Can you work these out from the model? Positions are in its coordinate system, mm. Round coordinates to 2 decimals unless told otherwise and drop trailing zeros. Answer in a Markdown table with one row per item. Add a question column.
(1) Suppose I cut it at A-A, the plane y = -7. Count the separate pieces of the cut face and the enclosed holes in it, then the cut area to 3 significant figures.
(2) If we mould it in two halves opening along X, with no side actions, what happens to faces 1 (the face through (-8.4, 7.8, 7)), 2 (the face through (-0.13, -14.96, 3.48))? For each: released by +X, released by -X, zero draft, split by the parting line, or undercut.
(3) I'm going to push flat-ended pins straight in: pin 1 (4 mm diameter, centred on y = 10, z = 6, fed in from +X); pin 2 (6 mm diameter, centred on x = -1.5, y = 6.5, fed in from +Z); pin 3 (4 mm diameter, centred on x = 16, z = 3.5, fed in from -Y); pin 4 (2 mm diameter, centred on y = -1.5, z = 2.5, fed in from -X). Where does each tip first touch, or does it pass through?
(4) If I drill on probe 1 along Y at (x, z) = (-24, 4.75) (3 decimals); probe 2 along X at (y, z) = (8.5, 3.25); probe 3 along X at (y, z) = (2.5, 6.75), over which ranges is the centre line in solid material (lowest first)?
from build123d import *

# Parameters (mm, degrees)
F1_DEPTH = 7
F2_R     = 6
F3_R     = 2


# Not quite as in the source:
# - a feature names something its author has since deleted; it is built from what else it names


with BuildPart() as f1:
    # F0 (on Top) → F1 (new body)
    with BuildSketch(Plane.XY):
        with BuildLine():
            ThreePointArc((-14.0623969756, 5.1112299037), (-13.1615738007, 7.1167868393), (-11.9765766631, 8.9686839202))
            ThreePointArc((-11.9765766631, 8.9686839202), (-39, 0), (-11.9765766631, -8.9686839202))
            ThreePointArc((-11.9765766631, -8.9686839202), (-13.1615738007, -7.1167868393), (-14.0623969756, -5.1112299037))
            ThreePointArc((-14.0623969756, -5.1112299037), (-35.175, 0), (-14.0623969756, 5.1112299037))
        make_face()
        with BuildLine():
            ThreePointArc((-9.9141796875, -5.1565168597), (-11.175, 0), (-9.9141796875, 5.1565168597))
            ThreePointArc((-9.9141796875, 5.1565168597), (-10.8069599633, 7.1374851726), (-11.9765766631, 8.9686839202))
            ThreePointArc((-11.9765766631, 8.9686839202), (-13.1615738007, 7.1167868393), (-14.0623969756, 5.1112299037))
            ThreePointArc((-14.0623969756, 5.1112299037), (-13.1387537824, 2.6294401687), (-12.825, 0))
            ThreePointArc((-12.825, 0), (-13.1387537824, -2.6294401687), (-14.0623969756, -5.1112299037))
            ThreePointArc((-14.0623969756, -5.1112299037), (-13.1615738007, -7.1167868393), (-11.9765766631, -8.9686839202))
            ThreePointArc((-11.9765766631, -8.9686839202), (-10.8069599633, -7.1374851726), (-9.9141796875, -5.1565168597))
        make_face()
        with BuildLine():
            ThreePointArc((-9.9141796875, 5.1565168597), (0, 11.175), (9.9141796875, 5.1565168597))
            ThreePointArc((9.9141796875, 5.1565168597), (10.8069599633, 7.1374851726), (11.9765766631, 8.9686839202))
            ThreePointArc((11.9765766631, 8.9686839202), (0, 14.9624757252), (-11.9765766631, 8.9686839202))
            ThreePointArc((-11.9765766631, 8.9686839202), (-10.8069599633, 7.1374851726), (-9.9141796875, 5.1565168597))
        make_face()
        with BuildLine():
            ThreePointArc((9.9141796875, 5.1565168597), (10.8552195512, 2.6542105222), (11.175, 0))
            ThreePointArc((11.175, 0), (10.8552195512, -2.6542105222), (9.9141796875, -5.1565168597))
            ThreePointArc((9.9141796875, -5.1565168597), (10.8069599633, -7.1374851726), (11.9765766631, -8.9686839202))
            ThreePointArc((11.9765766631, -8.9686839202), (13.1615738007, -7.1167868393), (14.0623969756, -5.1112299037))
            ThreePointArc((14.0623969756, -5.1112299037), (12.825, 0), (14.0623969756, 5.1112299037))
            ThreePointArc((14.0623969756, 5.1112299037), (13.1615738007, 7.1167868393), (11.9765766631, 8.9686839202))
            ThreePointArc((11.9765766631, 8.9686839202), (10.8069599633, 7.1374851726), (9.9141796875, 5.1565168597))
        make_face()
        with BuildLine():
            ThreePointArc((39, 0), (28.724862429, 14.2364207239), (11.9765766631, 8.9686839202))
            ThreePointArc((11.9765766631, 8.9686839202), (13.1615738007, 7.1167868393), (14.0623969756, 5.1112299037))
            ThreePointArc((14.0623969756, 5.1112299037), (26.6294401687, 10.8612462176), (35.175, 0))
            ThreePointArc((35.175, 0), (26.6294401687, -10.8612462176), (14.0623969756, -5.1112299037))
            ThreePointArc((14.0623969756, -5.1112299037), (13.1615738007, -7.1167868393), (11.9765766631, -8.9686839202))
            ThreePointArc((11.9765766631, -8.9686839202), (28.724862429, -14.2364207239), (39, 0))
        make_face()
        with BuildLine():
            ThreePointArc((11.9765766631, -8.9686839202), (10.8069599633, -7.1374851726), (9.9141796875, -5.1565168597))
            ThreePointArc((9.9141796875, -5.1565168597), (0, -11.175), (-9.9141796875, -5.1565168597))
            ThreePointArc((-9.9141796875, -5.1565168597), (-10.8069599633, -7.1374851726), (-11.9765766631, -8.9686839202))
            ThreePointArc((-11.9765766631, -8.9686839202), (0, -14.9624757252), (11.9765766631, -8.9686839202))
        make_face()
    extrude(amount=F1_DEPTH)

    # F2
    f2_edges = [f1.edges().sort_by_distance(p)[0] for p in [
        (-11.976577, -8.968684, 3.5),
        (11.976577, -8.968684, 3.5),
        (11.976577, 8.968684, 3.5),
        (-11.976577, 8.968684, 3.5),
    ]]
    fillet(f2_edges, radius=F2_R)

    # F3
    f3_edges = [f1.edges().sort_by_distance(p)[0] for p in [
        (-39, 0, 7),
        (-39, 0, 0),
    ]]
    fillet(f3_edges, radius=F3_R)


solid = f1.part
Calculated:
| question | item | result |
|---|---|---|
| 1 | separate pieces | 4 |
| 1 | enclosed holes | 0 |
| 1 | area | 152 mm² |
| 2 | face 1 | zero draft |
| 2 | face 2 | undercut |
| 3 | pin 1 | x = 36.58 |
| 3 | pin 2 | through |
| 3 | pin 3 | y = -13.75 |
| 3 | pin 4 | x = -38.99 |
| 4 | probe 1 | -15 to -11.175, 11.175 to 15 |
| 4 | probe 2 | -36.36 to -31.25, -16.75 to -7.25, 7.25 to 16.75, 31.25 to 36.36 |
| 4 | probe 3 | -37.74 to -34.89, -13.11 to -10.89, 10.89 to 13.11, 34.89 to 37.74 |
